```python
from build123d import *

# Parameters (mm, degrees)
PAD_DEPTH                  = 100
SKETCH001_R                = 6
POCKET_DEPTH               = 50.001
POCKETBODY_PITCH_ANGLE     = -90
POCKETBODY_PLACEMENT_ANGLE = -180


with BuildPart() as part:
    # Sketch → Pad (new body)
    with BuildSketch(Plane.XY):
        Polygon((0, 0), (0, 50), (6, 50), (6, 6), (50, 6), (50, 0), align=None)
    extrude(amount=PAD_DEPTH)

    # Sketch001 (on Face6 of Pad) → Pocket (cut, through all)
    with BuildSketch(Plane.XZ):
        with Locations((25, 50)):
            Circle(SKETCH001_R)
    extrude(amount=-POCKET_DEPTH, mode=Mode.SUBTRACT)


with BuildPart() as part_1:
    # PocketBody pitch: moved
    add(part.part.rotate(Axis((0, 0, 0), (0, 1, 0)), POCKETBODY_PITCH_ANGLE))


with BuildPart() as part_2:
    # PocketBody placement: moved
    add(part_1.part.moved(Location((-50, 50, 0))).rotate(Axis((-50, 50, 0), (0, 0, 1)), POCKETBODY_PLACEMENT_ANGLE))


solid = part_2.part
```
Here's how the part is built. I have some questions about the finished solid (model axes, mm). A direction names the side the tool comes from. Coordinates: 2 decimals unless noted, no trailing zeros. Order: outer loops, then holes, each group sorted by start corner. A loop starts at its lowest first (then second) coordinate and runs counter-clockwise, first axis right, second up.
1) Imagine slicing it at C-C on y = 14. List the corners of the cut face in (x, z) for me.
2) Imagine slicing it at A-A on x = 0. List the corners of the cut face in (y, z) for me.
3) Imagine slicing it at B-B on z = 25. List the corners of the cut face in (x, y) for me.
4) Imagine slicing it at D-D on z = 15.5. List the corners of the cut face in (x, y) for me, and give its area (3 significant figures).
5) Will these pins go through, and if not, where does the flat tip stop? pin 1 (1 mm diameter, centred on x = -6, z = 32.5, fed in from -Y); pin 2 (4 mm diameter, centred on y = 41, z = 29.5, fed in from +X).
6) Which directions (+Z, -Z, +X, -X, +Y, -Y) give clear straight access to the entire face, cutting with the end or side of a thin tool? Please do faces 1 (the face through (-1, 0, 3)), 2 (the face through (-1, 22, 6)).
7) We'd pull the mould along X, two halves only. Please class faces 3 (the face through (-1, 44, 33)), 4 (the face through (0, 47, 19)), 5 (the face through (50, 45, 14)): +X half, -X half, draft (parallel to the pull), parting line (faces both ways), or undercut.
8) I need wall thicknesses on line 1 (X direction, y = 46, z = 25); line 2 (Y direction, x = 32.5, z = 31); line 3 (Z direction, x = 7.5, y = 2.5). Which ranges of each line are inside material? Lowest first, please.
Response values:
1. outline: (-50, 0) - (50, 0) - (50, 6) - (-50, 6) - close
2. outline: (0, 0) - (50, 0) - (50, 19) - (44, 19) - (44, 6) - (0, 6) - close; (44, 31) - (50, 31) - (50, 50) - (44, 50) - close
3. outline: (-50, 44) - (-6, 44) - (-6, 50) - (-50, 50) - close; (6, 44) - (50, 44) - (50, 50) - (6, 50) - close
4. outline: (-50, 44) - (50, 44) - (50, 50) - (-50, 50) - close
4. area: 600 mm2
5. pin 1: stops at y = 44
5. pin 2: passes through
6. face 1: +Z, -Z, +X, -X, -Y
6. face 2: +Z, +X, -X, -Y
7. face 3: draft
7. face 4: undercut
7. face 5: +X half
8. line 1: x = -50 to -6, 6 to 50
8. line 2: y = 44 to 50
8. line 3: z = 0 to 6
